Geometry: final body of the model. Coordinates: model frame, mm. Face numbers are marked on the shaded views. A direction names the side the tool comes from. Give positions to 0.01 mm unless a question says otherwise; leave off trailing zeros. Order: outer loops, then holes, each group sorted by start corner. A loop starts at its lowest first (then second) coordinate and runs counter-clockwise, first axis right, second up. Notation, with made-up numbers: (2.25, 84.25) -> (59.25, 84.25) arc R22 cw to (59.25, 123.25) -> close; hole circle Ø9 at (22, 62). An arc over 180 degrees is marked (long way). One line per question, with ' | ' between items. Start each with the question number.
(1) First-contact query: pin 1 Ø1.4 at (x, y) = (1.5, -18) entering from -Z; pin 2 Ø1 at (x, z) = (21, 7.5) entering from +Y; pin 3 Ø3.5 at (y, z) = (-14.5, 9) entering from +X; pin 4 Ø2.5 at (x, y) = (35.15, 10.4) entering from +Z. Flat tips, straight axial feed; report the tip coordinate or a pass-through.
(2) Section C-C (z = 12.75). Return loops of the section in (x, y).
(3) Set-up query: the marked faces 1 and 2. Return all of +Z, -Z, +X, -X, +Y, -Y with unobstructed straight access to the full face (end or side cutting, diameter ignored); none if empty.
(4) Section D-D (x = -22.5). Return loops of the section in (y, z), then the cut area to 3 significant figures.
(5) Ray query, L1, parallel to X at y = -18, z = 7.75; L2, parallel to Y at x = 35.15, z = 0.45; L3, parallel to Y at x = -27, z = 1.1. Return the intervals inside material, ascending.
(6) Section A-A (x = -34.85). Return loops of the section in (y, z).
(7) Section B-B (y = 10.4). Return loops of the section in (x, z).
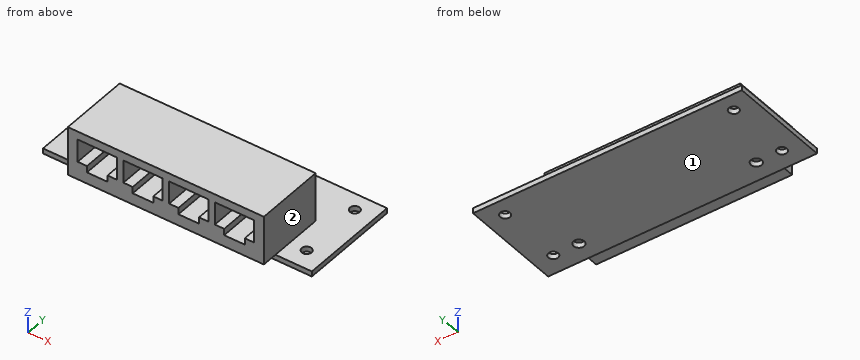
```python
from build123d import *

# Parameters (mm, degrees)
F0_W     = 82.3
F0_H     = 31.2
F0_R     = 1.5
F0_R_2   = 1.65
F1_DEPTH = 1.6
F2_W     = 60
F2_H     = 16.7
F2_R     = 1.65
F2_H_2   = 4.8
F3_DEPTH = 15
F4_W     = 6.3
F4_H     = 2
F5_DEPTH = 11


with BuildPart() as f1:
    # F0 (on Top) → F1 (new body)
    with BuildSketch(Plane.XY):
        Rectangle(F0_W, F0_H)
        with Locations((-34.85, -9.6)):
            Circle(F0_R, mode=Mode.SUBTRACT)
        with Locations((-27, -9.6)):
            Circle(F0_R_2, mode=Mode.SUBTRACT)
        with Locations((27.3, -9.6)):
            Circle(F0_R_2, mode=Mode.SUBTRACT)
        with Locations((35.15, -9.6)):
            Circle(F0_R, mode=Mode.SUBTRACT)
        with Locations((-34.85, 10.4)):
            Circle(F0_R, mode=Mode.SUBTRACT)
        with Locations((35.15, 10.4)):
            Circle(F0_R, mode=Mode.SUBTRACT)
    extrude(amount=F1_DEPTH)

    # F2 (on face) → F3 (join)
    with BuildSketch(Plane.XY.offset(1.6)):
        with Locations((0, -7.25)):
            Rectangle(F2_W, F2_H)
        with Locations((-27, -9.6)):
            Circle(F2_R, mode=Mode.SUBTRACT)
        with Locations((27.3, -9.6)):
            Circle(F2_R, mode=Mode.SUBTRACT)
        with Locations((0, -18)):
            Rectangle(F2_W, F2_H_2)
        with Locations((-27, -9.6)):
            Circle(F2_R)
        with Locations((27.3, -9.6)):
            Circle(F2_R)
    extrude(amount=F3_DEPTH)

    # F4 (on face) → F5 (cut)
    with BuildSketch(Plane.XZ.offset(20.4)):
        Polygon((-15, 14.1), (-27, 14.1), (-27, 7.1), (-24.1502, 7.1), (-17.8502, 7.1), (-15, 7.1), align=None)
        Polygon((-1, 14.1), (-13, 14.1), (-13, 7.1), (-10.1502, 7.1), (-3.8502, 7.1), (-1, 7.1), align=None)
        Polygon((13, 14.1), (1, 14.1), (1, 7.1), (3.8498, 7.1), (10.1498, 7.1), (13, 7.1), align=None)
        Polygon((27, 14.1), (15, 14.1), (15, 7.1), (17.8498, 7.1), (24.1498, 7.1), (27, 7.1), align=None)
        with Locations((20.9998, 6.1)):
            Rectangle(F4_W, F4_H)
        with Locations((6.9998, 6.1)):
            Rectangle(F4_W, F4_H)
        with Locations((-7.0002, 6.1)):
            Rectangle(F4_W, F4_H)
        with Locations((-21.0002, 6.1)):
            Rectangle(F4_W, F4_H)
    extrude(amount=-F5_DEPTH, mode=Mode.SUBTRACT)


solid = f1.part
```
Response:
1) pin 1: stops at z = 1.6 | pin 2: stops at y = 1.1 | pin 3: stops at x = 30 | pin 4: passes through
2) outline: (-30, -20.4) -> (-27, -20.4) -> (-27, -9.4) -> (-15, -9.4) -> (-15, -20.4) -> (-13, -20.4) -> (-13, -9.4) -> (-1, -9.4) -> (-1, -20.4) -> (1, -20.4) -> (1, -9.4) -> (13, -9.4) -> (13, -20.4) -> (15, -20.4) -> (15, -9.4) -> (27, -9.4) -> (27, -20.4) -> (30, -20.4) -> (30, 1.1) -> (-30, 1.1) -> close
3) face 1: -Z, +X, -X, +Y, -Y | face 2: +Z, +X, +Y, -Y
4) outline: (-20.4, 1.6) -> (-15.6, 1.6) -> (-15.6, 0) -> (15.6, 0) -> (15.6, 1.6) -> (1.1, 1.6) -> (1.1, 16.6) -> (-20.4, 16.6) -> (-20.4, 14.1) -> (-9.4, 14.1) -> (-9.4, 5.1) -> (-20.4, 5.1) -> close | area: 273 mm^2
5) L1: x = -30 to -27, -15 to -13, -1 to 1, 13 to 15, 27 to 30 | L2: y = -15.6 to -11.1, -8.1 to 8.9, 11.9 to 15.6 | L3: y = -15.6 to -11.25, -7.95 to 15.6
6) outline: (-15.6, 0) -> (-11.1, 0) -> (-11.1, 1.6) -> (-15.6, 1.6) -> close; (-8.1, 0) -> (8.9, 0) -> (8.9, 1.6) -> (-8.1, 1.6) -> close; (11.9, 0) -> (15.6, 0) -> (15.6, 1.6) -> (11.9, 1.6) -> close
7) outline: (-41.15, 0) -> (-36.35, 0) -> (-36.35, 1.6) -> (-41.15, 1.6) -> close; (-33.35, 0) -> (33.65, 0) -> (33.65, 1.6) -> (-33.35, 1.6) -> close; (36.65, 0) -> (41.15, 0) -> (41.15, 1.6) -> (36.65, 1.6) -> close
